Build history of the part. All positions in model axes, mm. Round coordinates to 2 decimals unless told otherwise and drop trailing zeros. One line per item, written item: value. Start each with the question number.
Item 1: Probe L1, parallel to Z at x = -165.1, y = 3.75; L2, parallel to X at y = 3.5, z = -44.45; L3, parallel to X at y = 1.5, z = -76.2. List the from-to ranges inside material, lowest first.
Item 2: Pin check, flat tip, straight feed: pin 1 (10 mm diameter, centred on x = 63.5, z = -76.2, fed in from -Y). Stop position of the tip, or through.
Item 3: Two-plate mould, pull along X, no slides. Class faces 1 (the cylindrical face through (107.9, 3.2, -77)), 2 (the flat face through (-2, 0, -2)): +X half, -X half, draft (parallel to the pull), parting line (faces both ways), or undercut.
```python
from build123d import *

# Parameters (mm, degrees)
SKETCH1_W             = 355.6
SKETCH1_H             = 254
BOSS_EXTRUDE1_DEPTH   = 6.35
SKETCH4_R             = 3.2639
CUT_EXTRUDE3_DEPTH    = 219.591313871
SKETCH5_R             = 6.35
SWITCH_MOUNTING_DEPTH = 219.591313871
SKETCH6_R             = 1.4605
CUT_EXTRUDE4_DEPTH    = 219.591313871
FILLET2_R             = 5.08


with BuildPart() as part:
    # Sketch1 → Boss-Extrude1 (new body)
    with BuildSketch(Plane(origin=(0, 0, 0), x_dir=(1, 0, 0), z_dir=(0, 1, 0))):
        Rectangle(SKETCH1_W, SKETCH1_H)
    extrude(amount=BOSS_EXTRUDE1_DEPTH)

    # Sketch4 → Cut-Extrude3 (cut, through all)
    with BuildSketch(Plane(origin=(0, 6.35, 0), x_dir=(1, 0, 0), z_dir=(0, 1, 0))):
        with Locations(Location((-165.1, 69.85, 0), (0, 0, 270))):
            Circle(SKETCH4_R)
        with Locations(Location((-165.1, 44.45, 0), (0, 0, 270))):
            Circle(SKETCH4_R)
        with Locations(Location((-165.1, -44.45, 0), (0, 0, 270))):
            Circle(SKETCH4_R)
        with Locations(Location((-165.1, -69.85, 0), (0, 0, 270))):
            Circle(SKETCH4_R)
        with Locations(Location((165.1, -69.85, 0), (0, 0, 90))):
            Circle(SKETCH4_R)
        with Locations(Location((165.1, -44.45, 0), (0, 0, 90))):
            Circle(SKETCH4_R)
        with Locations(Location((165.1, 44.45, 0), (0, 0, 90))):
            Circle(SKETCH4_R)
        with Locations(Location((165.1, 69.85, 0), (0, 0, 90))):
            Circle(SKETCH4_R)
    extrude(amount=-CUT_EXTRUDE3_DEPTH, mode=Mode.SUBTRACT)

    # Sketch5 → Switch Mounting (cut, through all)
    with BuildSketch(Plane(origin=(0, 6.35, 0), x_dir=(1, 0, 0), z_dir=(0, 1, 0))):
        with Locations(Location((25.4, 76.2, 0), (0, 0, 270))):
            Circle(SKETCH5_R)
        with Locations(Location((63.5, 76.2, 0), (0, 0, 270))):
            Circle(SKETCH5_R)
        with Locations(Location((101.6, 76.2, 0), (0, 0, 270))):
            Circle(SKETCH5_R)
    extrude(amount=-SWITCH_MOUNTING_DEPTH, mode=Mode.SUBTRACT)

    # Sketch6 → Cut-Extrude4 (cut, through all)
    with BuildSketch(Plane(origin=(0, 6.35, 0), x_dir=(1, 0, 0), z_dir=(0, 1, 0))):
        with Locations(Location((127, 76.2, 0), (0, 0, 270))):
            Circle(SKETCH6_R)
        with Locations(Location((0, 76.2, 0), (0, 0, 270))):
            Circle(SKETCH6_R)
    extrude(amount=-CUT_EXTRUDE4_DEPTH, mode=Mode.SUBTRACT)

    # Fillet2
    fillet2_edges = [part.edges().sort_by_distance(p)[0] for p in [
        (177.8, 3.175, 127),
        (-177.8, 3.175, 127),
        (-177.8, 3.175, -127),
        (177.8, 3.175, -127),
    ]]
    fillet(fillet2_edges, radius=FILLET2_R)


solid = part.part
```
Output:
1. L1: z = -127 to -73.11, -66.59 to -47.71, -41.19 to 41.19, 47.71 to 66.59, 73.11 to 127
1. L2: x = -177.8 to -168.36, -161.84 to 161.84, 168.36 to 177.8
1. L3: x = -177.8 to -1.46, 1.46 to 19.05, 31.75 to 57.15, 69.85 to 95.25, 107.95 to 125.54, 128.46 to 177.8
2. pin 1: passes through
3. face 1: undercut
3. face 2: draft
